```python
from build123d import *

# Parameters (mm, degrees)
SKETCH_1_W          = 80
SKETCH_1_H          = 125
SKETCH_1_R          = 12.5
EXTRUDE_1_DEPTH     = 5
SKETCH_2_W          = 28
SKETCH_2_H          = 18
CUT_EXTRUDE_1_DEPTH = 6
MM_CLEARANCE_1_D    = 4
MM_TRANSITIONAL_1_D = 5
FILLET_1_R          = 10
MM_TRANSITIONAL_2_D = 3
SKETCH_12_W         = 8
SKETCH_12_H         = 6
CUT_EXTRUDE_2_DEPTH = 6
FILLET_2_R          = 1


with BuildPart() as part:
    # 草图1 → 凸台-拉伸1 (new body)
    with BuildSketch(Plane(origin=(0, 0, 0), x_dir=(1, 0, 0), z_dir=(0, 1, 0))):
        with Locations((0, 2.5)):
            Rectangle(SKETCH_1_W, SKETCH_1_H)
        Circle(SKETCH_1_R, mode=Mode.SUBTRACT)
    extrude(amount=EXTRUDE_1_DEPTH)

    # 草图2 → 切除-拉伸1 (cut, through all)
    with BuildSketch(Plane(origin=(0, 5, 0), x_dir=(1, 0, 0), z_dir=(0, 1, 0))):
        with Locations((26, 56)):
            Rectangle(SKETCH_2_W, SKETCH_2_H)
    extrude(amount=-CUT_EXTRUDE_1_DEPTH, mode=Mode.SUBTRACT)

    # 大小mm Clearance 暗销孔1 (through all)
    with Locations(Plane(origin=(0, 5, 0), x_dir=(1, 0, 0), z_dir=(0, 1, 0))):
        with Locations((-23.5, -45), (23.5, -45), (28.5, 36), (-27.5, 41)):
            Hole(MM_CLEARANCE_1_D / 2)

    # 大小mm Transitional 暗销孔1 (through all)
    with Locations(Plane(origin=(0, 5, 0), x_dir=(1, 0, 0), z_dir=(0, 1, 0))):
        with Locations((0, -39), (0, 39)):
            Hole(MM_TRANSITIONAL_1_D / 2)

    # 圆角1
    fillet_1_edges = [part.edges().sort_by_distance(p)[0] for p in [
        (40, 2.5, -47),
        (-40, 2.5, -65),
        (40, 2.5, 60),
        (-40, 2.5, 60),
    ]]
    fillet(fillet_1_edges, radius=FILLET_1_R)

    # 大小mm Transitional 暗销孔2 (through all)
    with Locations(Plane(origin=(0, 5, 0), x_dir=(1, 0, 0), z_dir=(0, 1, 0))):
        with Locations((5.609431358, 33.8), (-18, 38.3)):
            Hole(MM_TRANSITIONAL_2_D / 2)

    # 草图12 → 切除-拉伸2 (cut, through all)
    with BuildSketch(Plane(origin=(0, 5, 0), x_dir=(1, 0, 0), z_dir=(0, 1, 0))):
        with Locations((16, 44)):
            Rectangle(SKETCH_12_W, SKETCH_12_H)
    extrude(amount=-CUT_EXTRUDE_2_DEPTH, mode=Mode.SUBTRACT)

    # 圆角2
    fillet_2_edges = [part.edges().sort_by_distance(p)[0] for p in [
        (12, 2.5, -41),
        (20, 2.5, -41),
        (12, 2.5, -65),
    ]]
    fillet(fillet_2_edges, radius=FILLET_2_R)


solid = part.part
```
Work out the finished part from the listing and answer in its coordinate system (mm). A direction names the side the tool comes from. Give positions to 0.01 mm unless a question says otherwise; leave off trailing zeros. Loops run counter-clockwise (first coordinate to the right, second up) from the corner with the lowest first, then second, coordinate; pieces in that order, holes last. Notation, with made-up numbers: (36.5, 54) - (40.5, 54) arc R30 ccw to (40.5, 93) - close; hole circle Ø1 at (-12, 17.25). An arc over 180 degrees is marked (long way). One line per question, with ' | ' between items.
(1) A tool of negligible diameter and unlimited length cuts with its end or side. For faces 5 (the face through (-9, 5, 11)), 6 (the face through (25, 3, -47)), 7 (the face through (12, 3, -53)), from which of +Z, -Z, +X, -X, +Y, -Y can it reach the whole face along a straight path? Write none if from no direction.
Recorded:
face 5: +Z, -Z, +X, -X, +Y | face 6: -Z, +X, +Y, -Y | face 7: -Z, +Y, -Y
(2) Each of these flat-tipped pins is pushed along its axis until it touches: pin 1 Ø1 at (x, y) = (31.5, 1) entering from -Z; pin 2 Ø1.5 at (x, y) = (17, 3) entering from -Z; pin 3 Ø1 at (x, y) = (27.5, 4.5) entering from -Z. Where does it stop, or does it pass through?
Recorded:
pin 1: stops at z = -46.95 | pin 2: stops at z = -41 | pin 3: stops at z = -47
(3) The part is cut by section D-D (x = -23.5). Write down the section's boundary in (y, z), then the cut area to 3 significant figures.
Recorded:
outline: (0, -65) - (5, -65) - (5, 43) - (0, 43) - close; (0, 47) - (5, 47) - (5, 60) - (0, 60) - close | area: 605 mm²
(4) The mould has two halves that part along X. Classify faces 1 (the face through (-40, 2, -2)), 2 (the face through (27.577, 2.465, -34.226)), 3 (the face through (0, 2, 60)), 4 (the face through (0.54, 2.47, -36.56)): +X half, -X half, draft (parallel to the pull), parting line (faces both ways), or undercut.
Recorded:
face 1: -X half | face 2: undercut | face 3: draft | face 4: undercut
(5) The part is cut by section A-A (y = 1.9). Count the separate pieces of the cut face and the enclosed holes in it, then the cut area to 3 significant figures.
Recorded:
separate pieces: 1 | enclosed holes: 9 | area: 8,770 mm²
(6) Straight lines are drawn through the part: probe 1 along X at (y, z) = (3.4, 45); probe 2 along Z at (x, y) = (0, 1.6); probe 3 along Z at (x, y) = (-27.5, 2.9). For each, find the intervals that lie inside material, in ascending order.
Recorded:
probe 1: x = -40 to -25.5, -21.5 to 21.5, 25.5 to 40 | probe 2: z = -65 to -41.5, -36.5 to -12.5, 12.5 to 36.5, 41.5 to 60 | probe 3: z = -65 to -43, -39 to 60
(7) The part is cut by section C-C (x = 0). Write down the section's boundary in (y, z), then the cut area to 3 significant figures.
Recorded:
outline: (0, -65) - (5, -65) - (5, -41.5) - (0, -41.5) - close; (0, -36.5) - (5, -36.5) - (5, -12.5) - (0, -12.5) - close; (0, 12.5) - (5, 12.5) - (5, 36.5) - (0, 36.5) - close; (0, 41.5) - (5, 41.5) - (5, 60) - (0, 60) - close | area: 450 mm²
(8) The part is cut by section B-B (x = 28.5). Write down the section's boundary in (y, z), then the cut area to 3 significant figures.
Recorded:
outline: (0, -47) - (5, -47) - (5, -38) - (0, -38) - close; (0, -34) - (5, -34) - (5, 60) - (0, 60) - close | area: 515 mm²
